from build123d import *

# Parameters (mm, degrees)
SKETCH1_W           = 48.26
SKETCH1_H           = 48.26
BOSS_EXTRUDE1_DEPTH = 6.35
CHAMFER1_SIZE       = 3.175
SKETCH4_W           = 28.575
SKETCH4_H           = 28.575
BOSS_EXTRUDE2_DEPTH = 12.7
CHAMFER2_SIZE       = 1.5875


with BuildPart() as part:
    # Sketch1 → Boss-Extrude1 (new body)
    with BuildSketch(Plane(origin=(0, 0, 0), x_dir=(1, 0, 0), z_dir=(0, 1, 0))):
        with Locations((24.13, 24.13)):
            Rectangle(SKETCH1_W, SKETCH1_H)
    extrude(amount=BOSS_EXTRUDE1_DEPTH)

    # Chamfer1
    chamfer1_edges = [part.edges().sort_by_distance(p)[0] for p in [
        (0, 3.175, -48.26),
        (48.26, 3.175, -48.26),
        (48.26, 3.175, 0),
        (0, 3.175, 0),
    ]]
    chamfer(chamfer1_edges, length=CHAMFER1_SIZE)

    # Sketch4 → Boss-Extrude2 (add)
    with BuildSketch(Plane.XZ):
        with Locations((24.13, -24.13)):
            Rectangle(SKETCH4_W, SKETCH4_H)
    extrude(amount=BOSS_EXTRUDE2_DEPTH)

    # Chamfer2
    chamfer2_edges = [part.edges().sort_by_distance(p)[0] for p in [
        (38.4175, 0, -24.13),
        (24.13, 0, -9.8425),
        (9.8425, 0, -24.13),
        (24.13, 0, -38.4175),
    ]]
    chamfer(chamfer2_edges, length=CHAMFER2_SIZE)


solid = part.part
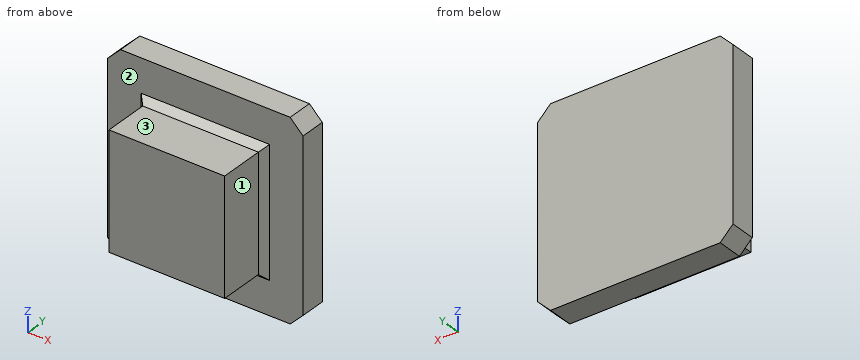
Geometry check sheet. Reference: the model listing, model coordinates, mm. Face numbers are marked on the shaded views. A direction names the side the tool comes from. Give positions to 0.01 mm unless a question says otherwise; leave off trailing zeros. Write each loop counter-clockwise with the first axis right and the second up, starting at its lowest first coordinate (ties: lowest second). Pieces come first, ordered by that corner, then holes. Notation, with made-up numbers: (87, -39.5) - (143, -39.5) arc R23 ccw to (143, -3.5) - close; hole circle Ø3 at (6.25, -13.75). An arc over 180 degrees is marked (long way). Put each result on its own line as item: value.
1. Sectioned sample at D-D, the plane z = -5. Enter the section's corners in (x, y).
Ans:
outline: (0, 0) - (48.26, 0) - (48.26, 6.35) - (0, 6.35) - close
2. Thickness scan on line 1 (X direction, y = -2.5, z = -31.5); line 2 (Z direction, x = 29, y = -10.75); line 3 (Y direction, x = 22.5, z = -40.5). Record the ranges inside material, lowest first.
Ans:
line 1: x = 9.84 to 38.42
line 2: z = -38.42 to -9.84
line 3: y = 0 to 6.35
3. Sectioned sample at C-C, the plane y = -5.25. Enter the section's corners in (x, z).
Ans:
outline: (9.84, -38.42) - (38.42, -38.42) - (38.42, -9.84) - (9.84, -9.84) - close
4. Go/stop test with flat-tipped pins: pin 1 (5 mm diameter, centred on x = 35.5, y = -6, fed in from -Z); pin 2 (5.5 mm diameter, centred on y = -10, z = -31, fed in from -X); pin 3 (9 mm diameter, centred on x = 25.5, y = -9.5, fed in from +Z). Record where each tip stops, or that it passes through.
Ans:
pin 1: stops at z = -38.42
pin 2: stops at x = 9.84
pin 3: stops at z = -9.84
5. Set-up check for the marked faces 1, 2 and 3: record each of +Z, -Z, +X, -X, +Y, -Y from which the full face is reachable in a straight line by a thin tool's end or side.
Ans:
face 1: +Z, -Z, +X, -Y
face 2: -Y
face 3: +Z, +X, -X, -Y
